Read the model definition and answer for the solid it produces. Units are mm, in the model's axes. Coordinates: 2 decimals unless noted, no trailing zeros. Loops run counter-clockwise (first coordinate to the right, second up) from the corner with the lowest first, then second, coordinate; pieces in that order, holes last. Notation, with made-up numbers: (-22, -37.75) -> (3, -37.75) arc R27 cw to (3, -14.75) -> close; hole circle Ø4 at (74, -11). An arc over 180 degrees is marked (long way). Answer as a JSON object with one key per item and string values. Group by question number.
1) Consider probe 1 along Z at (x, y) = (-58.5, -2); probe 2 along Z at (x, y) = (0, -2.35); probe 3 along Z at (x, y) = (117, -1.75). Determine where each line is inside the solid, lowest interval first. Write a range as [from, to].
2) Flat-ended cylindrical pins translate along their axes: P1, Ø22.5, axis at x = -58.5, z = -101.32, coming from the +Y side; P2, Ø1, axis at y = -3.5, z = -27, coming from the +X side. Find the tip coordinate at first contact, or state that the pin passes through.
3) Section B-B, the plane x = -57 is taken. Give the vertices of the cut face in (y, z), plus the area to 3 significant figures.
4) Section C-C, the plane z = -78 is taken. Give the vertices of the cut face in (x, y), plus the area to 3 significant figures.
5) Section D-D, the plane x = -27 is taken. Give the vertices of the cut face in (y, z), plus the area to 3 significant figures.
6) Section A-A, the plane z = 0 is taken. Give the vertices of the cut face in (x, y), plus the area to 3 significant figures.
from build123d import *

# Parameters (mm, degrees)
F0_R     = 130
F0_R_2   = 7
F0_R_3   = 87.5
F1_DEPTH = 5


with BuildPart() as f1:
    # F0 (on Front) → F1 (new body)
    with BuildSketch(Plane.XZ):
        Circle(F0_R)
        with Locations((-58.5, -101.324972)):
            Circle(F0_R_2, mode=Mode.SUBTRACT)
        with Locations((58.5, -101.324972)):
            Circle(F0_R_2, mode=Mode.SUBTRACT)
        with Locations((-117, 0)):
            Circle(F0_R_2, mode=Mode.SUBTRACT)
        with Locations((-58.5, 101.324972)):
            Circle(F0_R_2, mode=Mode.SUBTRACT)
        Circle(F0_R_3, mode=Mode.SUBTRACT)
        with Locations((117, 0)):
            Circle(F0_R_2, mode=Mode.SUBTRACT)
        with Locations((58.5, 101.324972)):
            Circle(F0_R_2, mode=Mode.SUBTRACT)
    extrude(amount=F1_DEPTH)


solid = f1.part
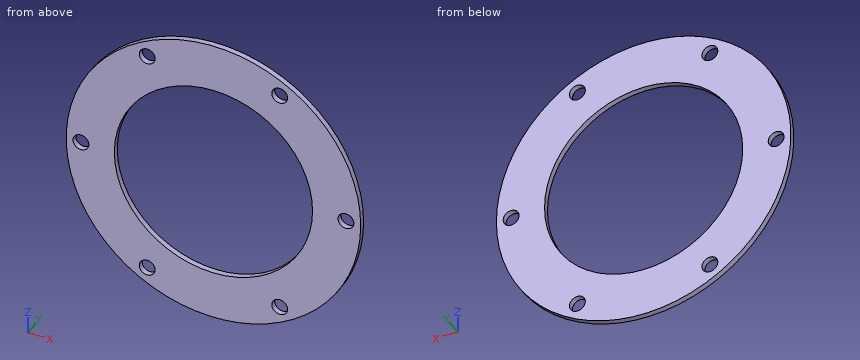
Determined:
{
 "1": {"probe 1": "[-116.09, -108.32], [-94.32, -65.07], [65.07, 94.32], [108.32, 116.09]", "probe 2": "[-130, -87.5], [87.5, 130]", "probe 3": "[-56.67, -7], [7, 56.67]"},
 "2": {"P1": "y = 0", "P2": "x = 127.27"},
 "3": {"outline": "(-5, -116.84) -> (0, -116.84) -> (0, -108.16) -> (-5, -108.16) -> close; (-5, -94.49) -> (0, -94.49) -> (0, -66.39) -> (-5, -66.39) -> close; (-5, 66.39) -> (0, 66.39) -> (0, 94.49) -> (-5, 94.49) -> close; (-5, 108.16) -> (0, 108.16) -> (0, 116.84) -> (-5, 116.84) -> close", "area": "368 mm²"},
 "4": {"outline": "(-104, -5) -> (-39.65, -5) -> (-39.65, 0) -> (-104, 0) -> close; (39.65, -5) -> (104, -5) -> (104, 0) -> (39.65, 0) -> close", "area": "643 mm²"},
 "5": {"outline": "(-5, -127.17) -> (0, -127.17) -> (0, -83.23) -> (-5, -83.23) -> close; (-5, 83.23) -> (0, 83.23) -> (0, 127.17) -> (-5, 127.17) -> close", "area": "439 mm²"},
 "6": {"outline": "(-130, -5) -> (-124, -5) -> (-124, 0) -> (-130, 0) -> close; (-110, -5) -> (-87.5, -5) -> (-87.5, 0) -> (-110, 0) -> close; (87.5, -5) -> (110, -5) -> (110, 0) -> (87.5, 0) -> close; (124, -5) -> (130, -5) -> (130, 0) -> (124, 0) -> close", "area": "285 mm²"}
}
